Read the model definition and answer for the solid it produces. Units are mm, in the model's axes. Face numbers are marked on the shaded views. Coordinates: 2 decimals unless noted, no trailing zeros. Write each loop counter-clockwise with the first axis right and the second up, starting at its lowest first coordinate (ties: lowest second). Pieces come first, ordered by that corner, then holes. Notation, with made-up numbers: (39.25, -34.5) -> (77.25, -34.5) arc R25 cw to (77.25, 2.5) -> close; hole circle Ø2 at (70, 88). An arc over 180 degrees is marked (long way). Write item = value, one per line. Start each with the question number.
1) Section A-A (y = 4) is taken. Determine the outline of the cut face in (x, z).
2) Find the intervals of material crossed by line 1 along X through (y, z) = (41, 10.5); line 2 along X through (y, z) = (49.5, 8.5); line 3 along Y through (x, z) = (28.5, 1.25), in increasing order. Write a range as from..to.
3) Section B-B (y = 110) is taken. Determine the outline of the cut face in (x, z), plus the area to 3 significant figures.
4) For a pull along Y with two mould halves and no side action, classify the marked faces 1, 2, 3 and 4 as released by +Y, released by -Y, zero draft, split by the parting line, or undercut.
5) Section C-C (x = 29.5) is taken. Determine the outline of the cut face in (y, z).
6) Section D-D (y = 26.5) is taken. Determine the outline of the cut face in (x, z), plus the area to 3 significant figures.
from build123d import *

# Parameters (mm, degrees)
SKETCH_6_W                  = 80
SKETCH_6_H                  = 150
EXTRUDE_1_DEPTH             = 12
SKETCH_8_R                  = 21
CUT_EXTRUDE_1_DEPTH         = 171.423003142
FILLET_1_R                  = 10
HOLE_WIZARD_M5_1_D          = 4.2
PATTERN_CIRCULAR_1_COUNT    = 4
CUT_EXTRUDE_2_DEPTH         = 171.423003142
CUT_EXTRUDE_3_DEPTH         = 5
FILLET_2_R                  = 3
PATTERN_LINEAR_1_COUNT      = 2
PATTERN_LINEAR_1_PITCH      = 28
PATTERN_LINEAR_1_COUNT_DIR2 = 2
PATTERN_LINEAR_1_PITCH_DIR2 = 50
HOLE_WIZARD_M6_1_AT_2_COUNT = 2
HOLE_WIZARD_M6_1_AT_2_PITCH = 98
HOLE_WIZARD_M6_1_AT_3_COUNT = 2
HOLE_WIZARD_M6_1_AT_3_PITCH = 126
HOLE_WIZARD_M5_2_D          = 4.2


with BuildPart() as part:
    # 草图6 → 凸台-拉伸1 (new body)
    with BuildSketch(Plane.XY):
        with Locations((40, 75)):
            Rectangle(SKETCH_6_W, SKETCH_6_H)
    extrude(amount=EXTRUDE_1_DEPTH)

    # 草图8 → 切除-拉伸1 (cut, through all)
    with BuildSketch(Plane.XY.offset(12)):
        with Locations((40, 30)):
            Circle(SKETCH_8_R)
    extrude(amount=-CUT_EXTRUDE_1_DEPTH, mode=Mode.SUBTRACT)

    # 圆角1
    fillet_1_edges = [part.edges().sort_by_distance(p)[0] for p in [
        (80, 0, 6),
        (0, 0, 6),
    ]]
    fillet(fillet_1_edges, radius=FILLET_1_R)

    # M5 螺纹孔1 (through all)
    with Locations(Plane.XY.offset(12)):
        with Locations((40, 56)):
            hole_wizard_m5_1 = Hole(HOLE_WIZARD_M5_1_D / 2)

    # 阵列(圆周)1: M5 螺纹孔1 ×4 about axis
    pattern_circular_1_axis = Axis((40, 30, 0), (0, 0, 1))
    for i in range(1, PATTERN_CIRCULAR_1_COUNT):
        add(hole_wizard_m5_1.rotate(pattern_circular_1_axis, i * 360 / PATTERN_CIRCULAR_1_COUNT), mode=Mode.SUBTRACT)

    # 草图11 → 切除-拉伸2 (cut, through all)
    with BuildSketch(Plane.XY.offset(12)):
        with BuildLine():
            Line((62.4, 68.414091782), (62.4, 73.414091782))
            ThreePointArc((62.4, 73.414091782), (65, 76.014091782), (67.6, 73.414091782))
            Line((67.6, 73.414091782), (67.6, 68.414091782))
            ThreePointArc((67.6, 68.414091782), (65, 65.814091782), (62.4, 68.414091782))
        make_face()
    cut_extrude_2 = extrude(amount=-CUT_EXTRUDE_2_DEPTH, mode=Mode.SUBTRACT)

    # 草图12 → 切除-拉伸3 (cut)
    with BuildSketch(Plane.XY.offset(12)):
        with BuildLine():
            Line((60.2, 68.414091782), (60.2, 73.414091782))
            ThreePointArc((60.2, 73.414091782), (65, 78.214091782), (69.8, 73.414091782))
            Line((69.8, 73.414091782), (69.8, 68.414091782))
            ThreePointArc((69.8, 68.414091782), (65, 63.614091782), (60.2, 68.414091782))
        make_face()
    cut_extrude_3 = extrude(amount=-CUT_EXTRUDE_3_DEPTH, mode=Mode.SUBTRACT)

    # 圆角2
    fillet_2_edges = [part.edges().sort_by_distance(p)[0] for p in [
        (0, 150, 6),
        (80, 150, 6),
    ]]
    fillet(fillet_2_edges, radius=FILLET_2_R)

    # 阵列(线性)1: 切除-拉伸2, Cut-Extrude 3 2 × 2
    with Locations(*[(-j * PATTERN_LINEAR_1_PITCH_DIR2, -i * PATTERN_LINEAR_1_PITCH, 0) for i in range(PATTERN_LINEAR_1_COUNT) for j in range(PATTERN_LINEAR_1_COUNT_DIR2) if (i, j) != (0, 0)]):
        add(cut_extrude_2, mode=Mode.SUBTRACT)
        add(cut_extrude_3, mode=Mode.SUBTRACT)

    # 草图13 → M6 螺纹孔1 (revolve, cut)
    with BuildSketch(Plane(origin=(70, 12, 12), x_dir=(0, -1, 0), z_dir=(1, 0, 0))):
        Polygon((0, 0), (0, 16.502151548), (2.5, 15), (2.5, 0), align=None)
    hole_wizard_m6_1 = revolve(axis=Axis((70, 12, 18.35), (0, 0, -1)), mode=Mode.SUBTRACT)

    # M6 螺纹孔1 at 2: M6 螺纹孔1 ×2
    with Locations(*[(0, i * HOLE_WIZARD_M6_1_AT_2_PITCH, 0) for i in range(1, HOLE_WIZARD_M6_1_AT_2_COUNT)]):
        add(hole_wizard_m6_1, mode=Mode.SUBTRACT)

    # M6 螺纹孔1 at 3: M6 螺纹孔1 ×2
    with Locations(*[(0, i * HOLE_WIZARD_M6_1_AT_3_PITCH, 0) for i in range(1, HOLE_WIZARD_M6_1_AT_3_COUNT)]):
        add(hole_wizard_m6_1, mode=Mode.SUBTRACT)

    # 镜向1: M6 螺纹孔1 across plane
    add(hole_wizard_m6_1.mirror(Plane.ZY.offset(-40)), mode=Mode.SUBTRACT)

    # 镜向1 copy 1 sketch → 镜向1 copy 1 (revolve, cut)
    with BuildSketch(Plane(origin=(10, 110, 12), x_dir=(0, -1, 0), z_dir=(-1, 0, 0))):
        Polygon((0, 0), (0, -16.502151548), (2.5, -15), (2.5, 0), align=None)
    revolve(axis=Axis((10, 110, 18.35), (0, 0, 1)), mode=Mode.SUBTRACT)

    # 镜向1 copy 2 sketch → 镜向1 copy 2 (revolve, cut)
    with BuildSketch(Plane(origin=(10, 138, 12), x_dir=(0, -1, 0), z_dir=(-1, 0, 0))):
        Polygon((0, 0), (0, -16.502151548), (2.5, -15), (2.5, 0), align=None)
    revolve(axis=Axis((10, 138, 18.35), (0, 0, 1)), mode=Mode.SUBTRACT)

    # M5 螺纹孔2 (through all)
    with Locations(Plane(origin=(0, 0, 0), x_dir=(-1, 0, 0), z_dir=(0, 0, -1))):
        with Locations((-12.5, 62.435602505), (-29.5, 62.435602505), (-29.5, 90.435602505), (-12.5, 90.435602505)):
            Hole(HOLE_WIZARD_M5_2_D / 2)


solid = part.part
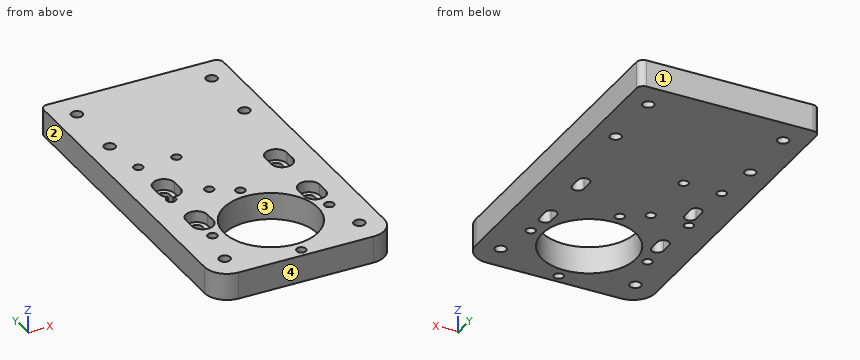
Answer key:
q1.outline = (2, 0) -> (37.9, 0) -> (37.9, 12) -> (2, 12) -> close; (42.1, 0) -> (78, 0) -> (78, 12) -> (42.1, 12) -> close
q2.line_1 = 0..10.2, 19.8..22.11, 57.89..60.2, 69.8..80
q2.line_2 = 0..12.48, 17.52..32.21, 47.79..62.48, 67.52..80
q2.line_3 = 0..12.43, 47.57..60.59, 64.28..88.59, 92.28..150
q3.outline = (0, 0) -> (7.5, 0) -> (7.5, 12) -> (0, 12) -> close; (12.5, 0) -> (67.5, 0) -> (67.5, 12) -> (12.5, 12) -> close; (72.5, 0) -> (80, 0) -> (80, 12) -> (72.5, 12) -> close
q3.area = 840 mm^2
q4.face_1 = released by +Y
q4.face_2 = zero draft
q4.face_3 = undercut
q4.face_4 = released by -Y
q5.outline = (0, 0) -> (11.81, 0) -> (11.81, 12) -> (0, 12) -> close; (48.19, 0) -> (60.34, 0) -> (60.34, 12) -> (48.19, 12) -> close; (64.54, 0) -> (88.34, 0) -> (88.34, 12) -> (64.54, 12) -> close; (92.54, 0) -> (150, 0) -> (150, 12) -> (92.54, 12) -> close
q6.outline = (0, 0) -> (19.29, 0) -> (19.29, 12) -> (0, 12) -> close; (60.71, 0) -> (80, 0) -> (80, 12) -> (60.71, 12) -> close
q6.area = 463 mm^2
